```python
from build123d import *

# Parameters (mm, degrees)
SKETCH1_W           = 14.6558
SKETCH1_H           = 7.9375
SKETCH1_W_2         = 1.5875
SKETCH1_H_2         = 4.7625
BOSS_EXTRUDE1_DEPTH = 3.175
SKETCH1_3_W         = 1.5875
SKETCH1_3_H         = 4.7625
BOSS_EXTRUDE2_DEPTH = 3.175
FILLET1_R           = 3.175


with BuildPart() as part:
    # Sketch1 → Boss-Extrude1 (new body)
    # profile 1 of 4: a face of its own
    with BuildSketch(Plane(origin=(0, 0, 0), x_dir=(1, 0, 0), z_dir=(0, 1, 0))):
        with Locations((7.3279, 3.96875)):
            Rectangle(SKETCH1_W, SKETCH1_H)
        with Locations((12.27455, 3.96875)):
            Rectangle(SKETCH1_W_2, SKETCH1_H_2, mode=Mode.SUBTRACT)
        with Locations((7.3279, 3.96875)):
            Rectangle(SKETCH1_W_2, SKETCH1_H_2, mode=Mode.SUBTRACT)
        with Locations((2.38125, 3.96875)):
            Rectangle(SKETCH1_W_2, SKETCH1_H_2, mode=Mode.SUBTRACT)
    # profile 2 of 4: a face of its own
    with BuildSketch(Plane(origin=(0, 0, 0), x_dir=(1, 0, 0), z_dir=(0, 1, 0))):
        with Locations((2.38125, 3.96875)):
            Rectangle(SKETCH1_W_2, SKETCH1_H_2)
    # profile 3 of 4: a face of its own
    with BuildSketch(Plane(origin=(0, 0, 0), x_dir=(1, 0, 0), z_dir=(0, 1, 0))):
        with Locations((7.3279, 3.96875)):
            Rectangle(SKETCH1_W_2, SKETCH1_H_2)
    # profile 4 of 4: a face of its own
    with BuildSketch(Plane(origin=(0, 0, 0), x_dir=(1, 0, 0), z_dir=(0, 1, 0))):
        with Locations((12.27455, 3.96875)):
            Rectangle(SKETCH1_W_2, SKETCH1_H_2)
    extrude(amount=-BOSS_EXTRUDE1_DEPTH)

    # Sketch1<3> → Boss-Extrude2 (add)
    with BuildSketch(Plane(origin=(0, 0, 0), x_dir=(1, 0, 0), z_dir=(0, 1, 0))):
        with Locations((2.38125, 3.96875)):
            Rectangle(SKETCH1_3_W, SKETCH1_3_H)
        with Locations((7.3279, 3.96875)):
            Rectangle(SKETCH1_3_W, SKETCH1_3_H)
        with Locations((12.27455, 3.96875)):
            Rectangle(SKETCH1_3_W, SKETCH1_3_H)
    extrude(amount=BOSS_EXTRUDE2_DEPTH)

    # Fillet1
    fillet1_edges = [part.edges().sort_by_distance(p)[0] for p in [
        (14.6558, -3.175, -3.96875),
        (7.3279, -3.175, -7.9375),
        (0, -3.175, -3.96875),
        (7.3279, -3.175, 0),
    ]]
    fillet(fillet1_edges, radius=FILLET1_R - 0.0001)  # a hair under: the kernel refuses the full size


solid = part.part
```
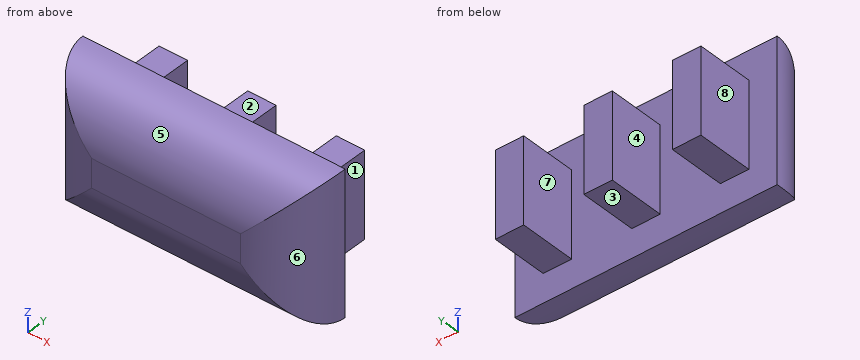
Source: CAD feature listing. Evaluate the final solid. Frame: model axes, mm. Face numbers are marked on the shaded views. A direction names the side the tool comes from. Round coordinates to 2 decimals unless told otherwise and drop trailing zeros. Order: outer loops, then holes, each group sorted by start corner. A loop starts at its lowest first (then second) coordinate and runs counter-clockwise, first axis right, second up. Notation, with made-up numbers: (86.5, -32.5) -> (135.5, -32.5) arc R19 ccw to (135.5, 3.5) -> close; hole circle Ø8 at (62, 69.25). An arc over 180 degrees is marked (long way). One line per item, written item: value. Start each with the question number.
Q1. Material intervals for probe 1 along X at (y, z) = (2.25, -3.5) (1 decimal); probe 2 along Z at (x, y) = (2.75, 0.75); probe 3 along Y at (x, z) = (4.25, -5.25), sorted ascending.
Q2. Access query for the marked faces 1, 2, 3 and 4. Directions: +Z, -Z, +X, -X, +Y, -Y. A direction counts if a zero-diameter tool reaches every point of the face in a straight line with its end or side. Return the directions, or none.
Q3. Section query D-D (y = -0.75). Return the cut outline in (x, z).
Q4. Pin query (flat end, axial travel): pin 1 (1 mm diameter, centred on y = 1, z = -4.5, fed in from +X); pin 2 (1.6 mm diameter, centred on y = 1, z = -4.5, fed in from -X); pin 3 (3 mm diameter, centred on x = 7.5, z = -2, fed in from -Y) (3 decimals); pin 4 (1.7 mm diameter, centred on x = 12, y = 1.5, fed in from +Z). Return the tip coordinate at first contact, or that it passes through.
Q5. Draft query along X for the marked faces 5, 6, 7 and 8. Return one class per face: pulls with the +X half, pulls with the -X half, needs draft (parallel to the pull), parting line crosses it, or undercut.
Q6. Section query A-A (y = 1.75). Give the number of separate pieces and of enclosed holes in the cut face, plus the area to 3 significant figures.
Findings below:
1. probe 1: 1.6 to 3.2, 6.5 to 8.1, 11.5 to 13.1
1. probe 2: -6.35 to -1.59
1. probe 3: -3.14 to 0
2. face 1: +Z, -Z, +X, +Y
2. face 2: +Z, +X, -X, +Y
2. face 3: -Z, +X, -X, +Y
2. face 4: +Z, -Z, +Y
3. outline: (0.09, -7.85) -> (14.57, -7.85) -> (14.57, -0.09) -> (0.09, -0.09) -> close
4. pin 1: x = 13.07
4. pin 2: x = 1.59
4. pin 3: y = -3.175
4. pin 4: z = -1.59
5. face 5: needs draft
5. face 6: pulls with the +X half
5. face 7: undercut
5. face 8: pulls with the -X half
6. separate pieces: 3
6. enclosed holes: 0
6. area: 22.7 mm²
